Could you check a few things on this model? Use its own coordinates, in mm. A direction names the side the tool comes from. Give positions to 0.01 mm unless a question says otherwise; leave off trailing zeros. Loops run counter-clockwise (first coordinate to the right, second up) from the corner with the lowest first, then second, coordinate; pieces in that order, holes last. Notation, with made-up numbers: M 2,69.5 L 55,69.5 A20 cw 55,83.5 Z; hole C 73.5,-17.5 d6. An arc over 180 degrees is marked long. Use a Markdown table: item, result. Add a question column.
1) Suppose I cut it at C-C on z = -20. List the corners of the cut face in (x, y) for me.
2) Suppose I cut it at D-D on y = 1. Count the separate pieces of the cut face and the enclosed holes in it, and give its area (3 significant figures).
3) Which directions (+Z, -Z, +X, -X, +Y, -Y) give clear straight access to the entire face, cutting with the end or side of a thin tool? Please do faces 4 (the flat face through (17, 0, 27)), 5 (the cylindrical face through (0, -4.9, -2.6)), 6 (the flat face through (-7, -5, -5)), 7 (the flat face through (-17, 0, -27)), 8 (the flat face through (11, 5, 13.5)).
4) Suppose I cut it at A-A on z = -11.5. List the corners of the cut face in (x, y) for me, and give its area (3 significant figures).
5) Will these pins go through, and if not, where does the flat tip stop? pin 1 Ø0.9 at (x, y) = (-11.5, 5.5) entering from -Z; pin 2 Ø6 at (x, y) = (-4.5, -3.5) entering from -Z; pin 3 Ø3.5 at (x, y) = (-11, 5.5) entering from +Z; pin 4 Ø0.8 at (x, z) = (-5, 27) entering from -Y.
6) We'd pull the mould along Z, two halves only. Please class faces 1 (the flat face through (6, -4, -5)), 2 (the flat face through (17.65, 5, -20)), 3 (the flat face through (-17, 5, -27.5)): +Z half, -Z half, draft (parallel to the pull), parting line (faces both ways), or undercut.
7) If I drill on line 1 along X through (y, z) = (7, 0); line 2 along Z through (x, y) = (17.5, 4); line 3 along Z through (x, y) = (-17.5, 4.25), over which ranges is the centre line in solid material (lowest first)? Write a range as [from, to].
8) Suppose I cut it at B-B on x = 2.5. List the corners of the cut face in (y, z) for me, and give its area (3 significant figures).
```python
from build123d import *

# Parameters (mm, degrees)
SKETCH_1_W          = 40000
SKETCH_1_H          = 55000
EXTRUDE_1_DEPTH     = 10000
SKETCH_2_R          = 6500
CUT_EXTRUDE_1_DEPTH = 17650
SKETCH_3_W          = 3000
SKETCH_3_H          = 1000
CUT_EXTRUDE_2_DEPTH = 35300
SKETCH_5_R          = 1600
CUT_EXTRUDE_4_DEPTH = 35300
SKETCH_7_R          = 4000
CUT_EXTRUDE_5_DEPTH = 100000
SCALE_1_SCALE       = 0.001
EXTRUDE_3_DEPTH     = 10
SKETCH_10_W         = 3
SKETCH_10_H         = 1.5
CUT_EXTRUDE_6_DEPTH = 10


with BuildPart() as part:
    # 草圖1 → 填料-伸長1 (new body)
    with BuildSketch(Plane(origin=(0, 0, 0), x_dir=(1, 0, 0), z_dir=(0, 1, 0))):
        Rectangle(SKETCH_1_W, SKETCH_1_H)
    extrude(amount=EXTRUDE_1_DEPTH)

    # 草圖2 → 除料-伸長1 (cut, symmetric)
    with BuildSketch(Plane(origin=(0, 0, 0), x_dir=(0, 0, -1), z_dir=(1, 0, 0))):
        with Locations((-20000, 0)):
            Circle(SKETCH_2_R)
        with Locations((20000, 0)):
            Circle(SKETCH_2_R)
    extrude(amount=CUT_EXTRUDE_1_DEPTH, both=True, mode=Mode.SUBTRACT)

    # 草圖3 → 除料-伸長2 (cut)
    with BuildSketch(Plane.XZ):
        with Locations((-11500, 27000)):
            Rectangle(SKETCH_3_W, SKETCH_3_H)
        with Locations((11500, 27000)):
            Rectangle(SKETCH_3_W, SKETCH_3_H)
        with Locations((11500, 13000)):
            Rectangle(SKETCH_3_W, SKETCH_3_H)
        with Locations((-11500, 13000)):
            Rectangle(SKETCH_3_W, SKETCH_3_H)
        with Locations((-11500, -13000)):
            Rectangle(SKETCH_3_W, SKETCH_3_H)
        with Locations((11500, -13000)):
            Rectangle(SKETCH_3_W, SKETCH_3_H)
        with Locations((11500, -27000)):
            Rectangle(SKETCH_3_W, SKETCH_3_H)
        with Locations((-11500, -27000)):
            Rectangle(SKETCH_3_W, SKETCH_3_H)
    extrude(amount=-CUT_EXTRUDE_2_DEPTH, mode=Mode.SUBTRACT)

    # 草圖5 → 除料-伸長4 (cut)
    with BuildSketch(Plane.XZ):
        with Locations(Location((-17500, 11500, 0), (0, 0, 270))):
            Circle(SKETCH_5_R)
        with Locations(Location((17500, 11500, 0), (0, 0, 270))):
            Circle(SKETCH_5_R)
        with Locations(Location((17500, -11500, 0), (0, 0, 270))):
            Circle(SKETCH_5_R)
        with Locations(Location((-17500, -11500, 0), (0, 0, 270))):
            Circle(SKETCH_5_R)
        with Locations(Location((0, 11500, 0), (0, 0, 270))):
            Circle(SKETCH_5_R)
        with Locations(Location((0, 0, 0), (0, 0, 270))):
            Circle(SKETCH_5_R)
        with Locations(Location((0, -11500, 0), (0, 0, 270))):
            Circle(SKETCH_5_R)
        with Locations(Location((-17500, 0, 0), (0, 0, 270))):
            Circle(SKETCH_5_R)
        with Locations(Location((17500, 0, 0), (0, 0, 270))):
            Circle(SKETCH_5_R)
    extrude(amount=-CUT_EXTRUDE_4_DEPTH, mode=Mode.SUBTRACT)

    # 草圖7 → 除料-伸長5 (cut)
    with BuildSketch(Plane(origin=(20000, 0, 0), x_dir=(0, 0, -1), z_dir=(1, 0, 0))):
        with Locations((20000, 0)):
            Circle(SKETCH_7_R)
        with Locations((-20000, 0)):
            Circle(SKETCH_7_R)
    extrude(amount=-CUT_EXTRUDE_5_DEPTH, mode=Mode.SUBTRACT)


with BuildPart() as part_1:
    # 縮放比例1: scaled about (0, 0, 0)
    add(part.part.scale(SCALE_1_SCALE))

    # 草圖9 → 填料-伸長3 (add)
    with BuildSketch(Plane.XZ):
        with BuildLine():
            Line((-15, -2), (-1.661324773, -2))
            ThreePointArc((-1.661324773, -2), (0, -2.6), (1.661324773, -2))
            Line((1.661324773, -2), (15, -2))
            Line((15, -2), (15, -8))
            Line((15, -8), (-15, -8))
            Line((-15, -8), (-15, -2))
        make_face()
    extrude(amount=EXTRUDE_3_DEPTH)

    # 草圖10 → 除料-伸長6 (cut)
    with BuildSketch(Plane(origin=(0, 0, -8), x_dir=(-1, 0, 0), z_dir=(0, 0, -1))):
        with Locations((-7.5, -4.25)):
            Rectangle(SKETCH_10_W, SKETCH_10_H)
        with Locations((7.5, -4.25)):
            Rectangle(SKETCH_10_W, SKETCH_10_H)
    extrude(amount=-CUT_EXTRUDE_6_DEPTH, mode=Mode.SUBTRACT)


solid = part_1.part
```
Answer block:
| question | item | result |
|---|---|---|
| 1 | outline | M -20,4 L -17.65,4 L -17.65,6.5 L 17.65,6.5 L 17.65,4 L 20,4 L 20,10 L -20,10 Z |
| 2 | separate pieces | 3 |
| 2 | enclosed holes | 13 |
| 2 | area | 1,120 mm^2 |
| 3 | face 4 | +Z, +X, -X, -Y |
| 3 | face 5 | +Z, -Y |
| 3 | face 6 | +Z, -Z |
| 3 | face 7 | -Z, +X, -X, -Y |
| 3 | face 8 | +Y, -Y |
| 4 | outline | M -20,0 L -19.1,0 L -19.1,10 L -20,10 Z; M -15.9,0 L -1.6,0 L -1.6,10 L -15.9,10 Z; M 1.6,0 L 15.9,0 L 15.9,10 L 1.6,10 Z; M 19.1,0 L 20,0 L 20,10 L 19.1,10 Z |
| 4 | area | 304 mm^2 |
| 5 | pin 1 | stops at z = -26.5 |
| 5 | pin 2 | stops at z = -8 |
| 5 | pin 3 | stops at z = 27.5 |
| 5 | pin 4 | stops at y = 0 |
| 6 | face 1 | draft |
| 6 | face 2 | undercut |
| 6 | face 3 | -Z half |
| 7 | line 1 | x = [-20, -19.1], [-15.9, -1.6], [1.6, 15.9], [19.1, 20] |
| 7 | line 2 | z = [-27.5, -25.12], [-14.88, -13.1], [-9.9, -1.6], [1.6, 9.9], [13.1, 14.88], [25.12, 27.5] |
| 7 | line 3 | z = [-27.5, -24.92], [-15.08, -13.1], [-9.9, -1.6], [1.6, 9.9], [13.1, 15.08], [24.92, 27.5] |
| 8 | outline | M -10,-8 L 0,-8 L 0,-13.5 A6.5 cw 0,-26.5 L 0,-27.5 L 10,-27.5 L 10,27.5 L 0,27.5 L 0,26.5 A6.5 cw 0,13.5 L 0,-2 L -10,-2 Z |
| 8 | area | 477 mm^2 |
